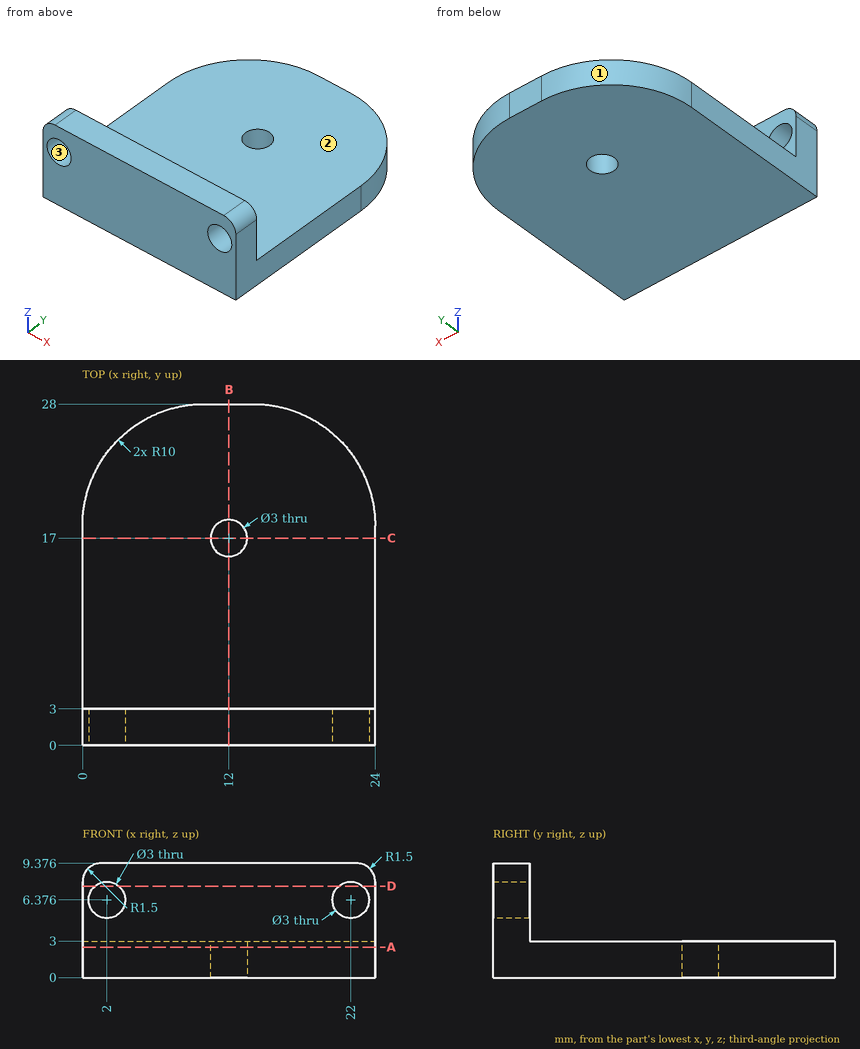
Source: three-view drawing plus pictorial views. Frame: mm from the lowest corner of the part. Round coordinates to 2 decimals unless told otherwise and drop trailing zeros. Write each loop counter-clockwise with the first axis right and the second up, starting at its lowest first coordinate (ties: lowest second). Pieces come first, ordered by that corner, then holes. Notation, with made-up numbers: M 38.25,39.5 L 73.25,39.5 A17 ccw 73.25,63.5 Z; hole C 68.25,-27.75 d4. An arc over 180 degrees is marked long. Use CSV: the item, a comma, the result in double quotes. Start each with the question number.
Q1. First-contact query: P1, Ø1.8, axis at x = 22, z = 6.38, coming from the -Y side; P2, Ø5, axis at x = 2, z = 6.38, coming from the +Y side; P3, Ø2, axis at x = 19, y = 11, coming from the +Z side; P4, Ø3, axis at y = 20.5, z = 2.5, coming from the +X side. Flat tips, straight axial feed; report the tip coordinate or a pass-through.
Q2. Cut plane B-B on x = 12. Output: boundary loops of the cut face in (y, z).
Q3. Cut plane D-D on z = 7.5. Output: boundary loops of the cut face in (x, y).
Q4. Line query: line 1 (Y direction, x = 12, z = 1.05); line 2 (Y direction, x = 16.5, z = 7.25). Output: solid intervals per line, ascending. Write a range as from..to.
Q5. Cut plane C-C on y = 17. Output: boundary loops of the cut face in (x, z), plus the area to 3 significant figures.
Q6. Pull-direction query (X, two-part tool) for the marked faces 1, 2 and 3; classes: +X half, -X half, draft (parallel to the pull), parting line (faces both ways), or undercut.
Q7. Cut plane A-A on z = 2.5. Output: boundary loops of the cut face in (x, y).
Results found:
1,P1,"through"
1,P2,"y = 3"
1,P3,"z = 3"
1,P4,"x = 23.95"
2,outline,"M 0,0 L 15.5,0 L 15.5,3 L 3,3 L 3,9.38 L 0,9.38 Z; M 18.5,0 L 28,0 L 28,3 L 18.5,3 Z"
3,outline,"M 0,0 L 1.01,0 L 1.01,3 L 0,3 Z; M 2.99,0 L 21.01,0 L 21.01,3 L 2.99,3 Z; M 22.99,0 L 24,0 L 24,3 L 22.99,3 Z"
4,line 1,"0..15.5, 18.5..28"
4,line 2,"0..3"
5,outline,"M 0,0 L 10.5,0 L 10.5,3 L 0,3 Z; M 13.5,0 L 24,0 L 24,3 L 13.5,3 Z"
5,area,"63.0 mm^2"
6,face 1,"-X half"
6,face 2,"draft"
6,face 3,"undercut"
7,outline,"M 0,0 L 24,0 L 24,18 A10 ccw 14,28 L 10,28 A10 ccw 0,18 Z; hole C 12,17 d3"
